The listing builds one solid part. Answer for the finished solid, in the listing's coordinates (mm). Face numbers are marked on the shaded views. Round coordinates to 2 decimals unless told otherwise and drop trailing zeros. Write each loop counter-clockwise with the first axis right and the second up, starting at its lowest first coordinate (ties: lowest second). Pieces come first, ordered by that corner, then holes.
Item 1: Each of these flat-tipped pins is pushed along its axis until it touches: pin 1 (6 mm diameter, centred on x = 26.5, z = -0.5, fed in from +Y); pin 2 (3 mm diameter, centred on y = 1.5, z = -0.5, fed in from -X); pin 3 (2 mm diameter, centred on y = -6.5, z = -3, fed in from +X). Where does it stop, or does it pass through?
Item 2: Find section B-B on x = 36. Give the vertices of the cut face in (y, z).
Item 3: For a pull along Y with two mould halves and no side action, classify the marked faces 1, 2 and 3 as +Y half, -Y half, draft (parallel to the pull), parting line (faces both ways), or undercut.
Item 4: Find section C-C on y = 9.5. Give the vertices of the cut face in (x, z).
Item 5: Find section A-A on z = -11. Give the vertices of the cut face in (x, y) (1 decimal), then the cut area to 3 significant figures.
Item 6: Find the intervals of material crossed by probe 1 along X at (y, z) = (-9, -12); probe 2 along X at (y, z) = (-13, 7.5); probe 3 along Y at (x, z) = (6, -10), in increasing order.
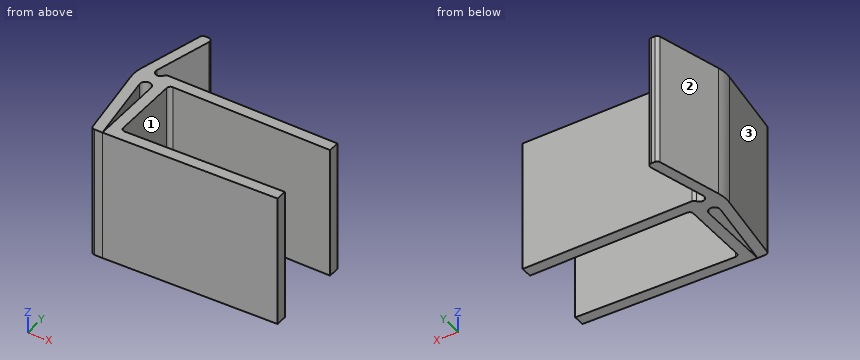
```python
from build123d import *

# Parameters (mm, degrees)
F1_DEPTH      = 18
F1_DEPTH_BACK = 18
F3_DEPTH      = 18
F3_DEPTH_BACK = 18
F4_R          = 1
F5_R          = 10
F6_R          = 1


with BuildPart() as f1:
    # F0 (on Top) → F1 (new body, two sides)
    with BuildSketch(Plane.XY) as f1_sk:
        Polygon((0, 0), (44, 0), (44, 3), (-3, 3), (-3, -23.081818), (44, -21.8), (44, -18.8), (0, -20), align=None)
    extrude(amount=F1_DEPTH)
    extrude(f1_sk.sketch, amount=-F1_DEPTH_BACK)

    # F2 (on Top) → F3 (join, two sides)
    with BuildSketch(Plane.XY) as f3_sk:
        with BuildLine():
            ThreePointArc((-3, 3), (-4.472403, 1.708738), (-5.560431, 3.337087))
            Line((-5.560431, 3.337087), (-1.095617, 20))
            Line((-1.095617, 20), (-4.095617, 20))
            Line((-4.095617, 20), (-9.454601, 0))
            Line((-9.454601, 0), (-6.005, -23.081818))
            Line((-6.005, -23.081818), (-3.005, -23.081818))
            Line((-3.005, -23.081818), (-5.973227, -3.220949))
            ThreePointArc((-5.973227, -3.220949), (-4.605602, -1.509287), (-3, -3))
            Line((-3, -3), (-3, 3))
        make_face()
    extrude(amount=F3_DEPTH)
    extrude(f3_sk.sketch, amount=-F3_DEPTH_BACK)

    # F4
    f4_edges = [f1.edges().sort_by_distance(p)[0] for p in [
        (-4.095617, 20, 0),
        (-1.095617, 20, 0),
        (-3, 3, 0),
        (-6.005, -23.081818, 0),
    ]]
    fillet(f4_edges, radius=F4_R)

    # F5
    f5_edges = [f1.edges().sort_by_distance(p)[0] for p in [
        (-9.454601, 0, 0),
    ]]
    fillet(f5_edges, radius=F5_R)

    # F6
    f6_edges = [f1.edges().sort_by_distance(p)[0] for p in [
        (0, 0, 0),
        (0, -20, 0),
    ]]
    fillet(f6_edges, radius=F6_R)


solid = f1.part
```
Check values:
1. pin 1: stops at y = 3
1. pin 2: stops at x = -9.24
1. pin 3: stops at x = 0
2. outline: (-22.02, -18) - (-19.02, -18) - (-19.02, 18) - (-22.02, 18) - close; (0, -18) - (3, -18) - (3, 18) - (0, 18) - close
3. face 1: undercut
3. face 2: +Y half
3. face 3: -Y half
4. outline: (-6.91, -18) - (-3.91, -18) - (-3.91, 18) - (-6.91, 18) - close
5. outline: (-9.1, -2.1) - (-6.1, -22.2) arc R1 ccw to (-5.1, -23.1) - (-3, -23.1) - (-6, -3.2) arc R1.5 cw (long way) to (-3, -3) - (-3, -23.1) - (44, -21.8) - (44, -18.8) - (1, -20) arc R1 cw to (0, -19) - (0, -1) arc R1 cw to (1, 0) - (44, 0) - (44, 3) - (-2.2, 3) arc R1 ccw to (-3.1, 2.4) arc R1.3 cw to (-5.6, 3.3) - (-1.4, 18.7) arc R1 ccw to (-2.4, 20) - (-3.3, 20) arc R1 ccw to (-4.3, 19.3) - (-8.9, 2) arc R10 ccw to start
5. area: 483 mm2
6. probe 1: x = -8.11 to -5.11, -3 to 0
6. probe 2: x = -7.51 to -4.51, -3 to 0
6. probe 3: y = -22.84 to -19.84, 0 to 3
